Model file for the job. Use its own axes, mm. Face numbers are marked on the shaded views. A direction names the side the tool comes from. Give positions to 0.01 mm unless a question says otherwise; leave off trailing zeros. Use CSV: the item, a comma, the result in double quotes. Start each with the question number.
(1) Pull direction Z, two halves, no side cores. Call the marked faces 1, 2 and 3: pulls with the +Z half, pulls with the -Z half, needs draft (parallel to the pull), parting line crosses it, or undercut.
(2) Drill centre lines: probe 1 along X at (y, z) = (-3, -3.5); probe 2 along X at (y, z) = (-3.75, 0); probe 3 along Z at (x, y) = (12.5, -5.5). Where is each one in solid material? Low to high.
(3) Cut at A-A on y = -5. State how many separate pieces and enclosed holes the cut face has, then the cut area to 3 significant figures.
(4) Flat gauge pins, fed straight in: pin 1 (4 mm diameter, centred on y = -6.5, z = -16, fed in from +X); pin 2 (2.5 mm diameter, centred on y = -4.5, z = 16.5, fed in from -X); pin 3 (3 mm diameter, centred on y = -3, z = 21, fed in from +X). Where does each tip first touch, or does it go through?
(5) 3-axis set-ups, long thin cutter, end or side, ignore diameter. For the marked faces 4 and 5: which of +Z, -Z, +X, -X, +Y, -Y reach the whole face in a straight line?
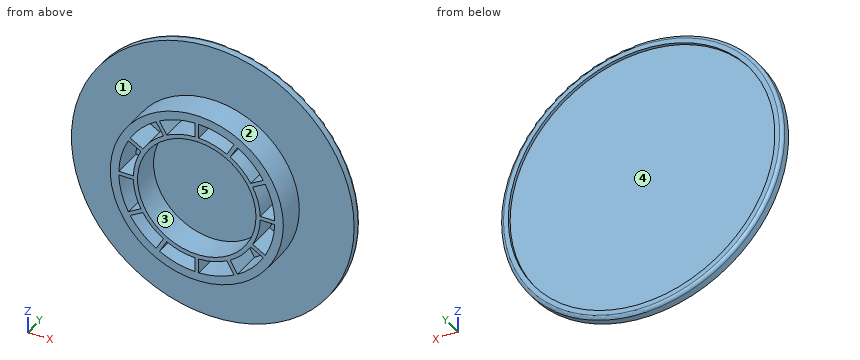
from build123d import *

# Parameters (mm, degrees)
FILLET1_R          = 0.762
SKETCH2_R          = 31.623
CUT_EXTRUDE1_DEPTH = 0.762
CUT_EXTRUDE2_DEPTH = 7.112
CIRPATTERN1_COUNT  = 12


with BuildPart() as part:
    # Sketch1 → Revolve1 (revolve)
    with BuildSketch(Plane.XY):
        Polygon((0, 0), (33.528, 0), (33.528, -2.3495), (20.5232, -2.3495), (20.5232, -9.017), (14.0462, -9.017), (14.0462, -2.3495), (0, -2.3495), align=None)
    revolve(axis=Axis((0, 0, 0), (0, 1, 0)))

    # Fillet1
    fillet1_edges = [part.edges().sort_by_distance(p)[0] for p in [
        (-33.528, 0, 0),
    ]]
    fillet(fillet1_edges, radius=FILLET1_R)

    # Sketch2 → Cut-Extrude1 (cut)
    with BuildSketch(Plane(origin=(0, 0, 0), x_dir=(1, 0, 0), z_dir=(0, 1, 0))):
        Circle(SKETCH2_R)
    extrude(amount=-CUT_EXTRUDE1_DEPTH, mode=Mode.SUBTRACT)

    # Sketch3 → Cut-Extrude2 (cut)
    with BuildSketch(Plane.XZ.offset(9.017)):
        with BuildLine():
            Line((-8.846826654, 16.237553251), (-7.131682909, 13.266837141))
            ThreePointArc((-7.131682909, 13.266837141), (-3.898384221, 14.548967981), (-0.4572, 15.055259446))
            Line((-0.4572, 15.055259446), (-0.4572, 18.485546938))
            ThreePointArc((-0.4572, 18.485546938), (-4.785874727, 17.861127639), (-8.846826654, 16.237553251))
        make_face()
    cut_extrude2 = extrude(amount=-CUT_EXTRUDE2_DEPTH, mode=Mode.SUBTRACT)

    # CirPattern1: Cut-Extrude2 ×12 about axis
    cirpattern1_axis = Axis((0, 0, 0), (0, 1, 0))
    for i in range(1, CIRPATTERN1_COUNT):
        add(cut_extrude2.rotate(cirpattern1_axis, i * 360 / CIRPATTERN1_COUNT), mode=Mode.SUBTRACT)


solid = part.part
Check result:
1,face 1,"needs draft"
1,face 2,"parting line crosses it"
1,face 3,"undercut"
2,probe 1,"-20.22 to -18.16, -14.65 to -13.6, 13.6 to 14.65, 18.16 to 20.22"
2,probe 2,"-20.52 to -14.05, 14.05 to 20.52"
2,probe 3,"-16.28 to -13.63, -8.4 to -6.41, 6.41 to 8.4, 13.63 to 16.28"
3,separate pieces,"1"
3,enclosed holes,"13"
3,area,"380 mm²"
4,pin 1,"x = 15.01"
4,pin 2,"x = -13.73"
4,pin 3,"x = 27.17"
5,face 4,"+Y"
5,face 5,"-Y"
